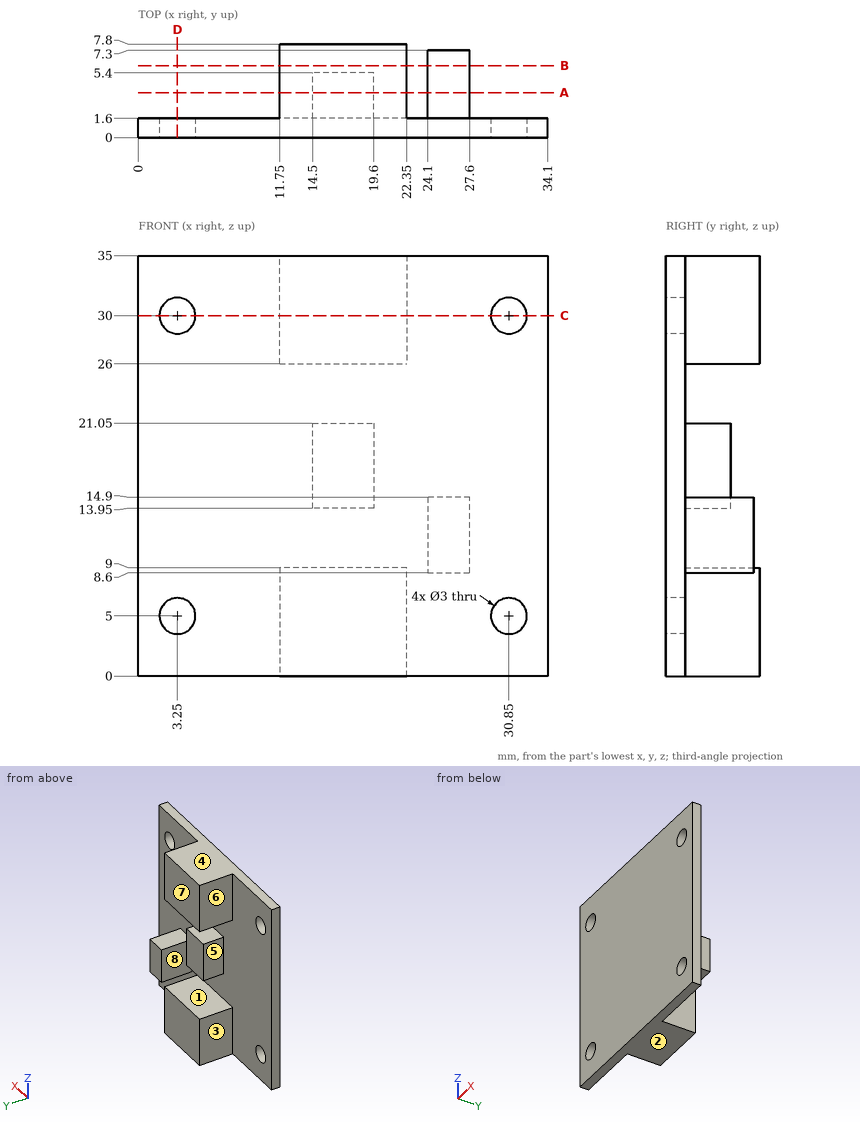
The figure shows three views and two pictorial views of one solid part (mm, origin at its lowest corner). Answer the questions. A direction names the side the tool comes from. Round coordinates to 2 decimals unless told otherwise and drop trailing zeros. Order: outer loops, then holes, each group sorted by start corner. A loop starts at its lowest first (then second) coordinate and runs counter-clockwise, first axis right, second up.
Q1. Find the intervals of material crossed by line 1 along Z through (x, y) = (30.85, 0.5); line 2 along X through (y, z) = (0.65, 30); line 3 along Z through (x, y) = (19, 7.25), in increasing order.
Solution:
line 1: z = 0 to 3.5, 6.5 to 28.5, 31.5 to 35
line 2: x = 0 to 1.75, 4.75 to 29.35, 32.35 to 34.1
line 3: z = 0 to 9, 26 to 35
Q2. Given pin 1 Ø5 at (x, z) = (30.85, 5) entering from +Y; pin 2 Ø1.9 at (y, z) = (4, 17.5) entering from +X; pin 3 Ø3 at (x, z) = (25.5, 10.5) entering from +Y, each flat-ended and moving along its own axis, determine where each tip first touches the part or whether it passes through.
Solution:
pin 1: stops at y = 1.6
pin 2: stops at x = 19.6
pin 3: stops at y = 7.3
Q3. A tool of negligible diameter and unlimited length cuts with its end or side. For the marked faces 4, 5, 6, 7 and 8, from which of +Z, -Z, +X, -X, +Y, -Y can it reach the whole face along a straight path? Write none if from no direction.
Solution:
face 4: +Z, +X, -X, +Y, -Y
face 5: -X, +Y
face 6: +Z, -Z, -X, +Y
face 7: +Z, -Z, +X, -X, +Y
face 8: +Z, -Z, +Y
Q4. The mould has two halves that part along Z. Classify the marked faces 1, 2 and 3: pulls with the +Z half, pulls with the -Z half, needs draft (parallel to the pull), parting line crosses it, or undercut.
Solution:
face 1: undercut
face 2: pulls with the -Z half
face 3: needs draft
Q5. A cutting plane is placed at D-D, the plane x = 3.25. Determine the outline of the cut face in (y, z).
Solution:
outline: (0, 0) - (1.6, 0) - (1.6, 3.5) - (0, 3.5) - close; (0, 6.5) - (1.6, 6.5) - (1.6, 28.5) - (0, 28.5) - close; (0, 31.5) - (1.6, 31.5) - (1.6, 35) - (0, 35) - close
Q6. A cutting plane is placed at B-B, the plane y = 6. Determine the outline of the cut face in (x, z), then the cut area to 3 significant figures.
Solution:
outline: (11.75, 0) - (22.35, 0) - (22.35, 9) - (11.75, 9) - close; (11.75, 26) - (22.35, 26) - (22.35, 35) - (11.75, 35) - close; (24.1, 8.6) - (27.6, 8.6) - (27.6, 14.9) - (24.1, 14.9) - close
area: 213 mm2
Q7. A cutting plane is placed at A-A, the plane y = 3.75. Determine the outline of the cut face in (x, z).
Solution:
outline: (11.75, 0) - (22.35, 0) - (22.35, 9) - (11.75, 9) - close; (11.75, 26) - (22.35, 26) - (22.35, 35) - (11.75, 35) - close; (14.5, 13.95) - (19.6, 13.95) - (19.6, 21.05) - (14.5, 21.05) - close; (24.1, 8.6) - (27.6, 8.6) - (27.6, 14.9) - (24.1, 14.9) - close
Q8. A cutting plane is placed at C-C, the plane z = 30. Determine the outline of the cut face in (x, y), then the cut area to 3 significant figures.
Solution:
outline: (0, 0) - (1.75, 0) - (1.75, 1.6) - (0, 1.6) - close; (4.75, 0) - (29.35, 0) - (29.35, 1.6) - (22.35, 1.6) - (22.35, 7.8) - (11.75, 7.8) - (11.75, 1.6) - (4.75, 1.6) - close; (32.35, 0) - (34.1, 0) - (34.1, 1.6) - (32.35, 1.6) - close
area: 111 mm2
